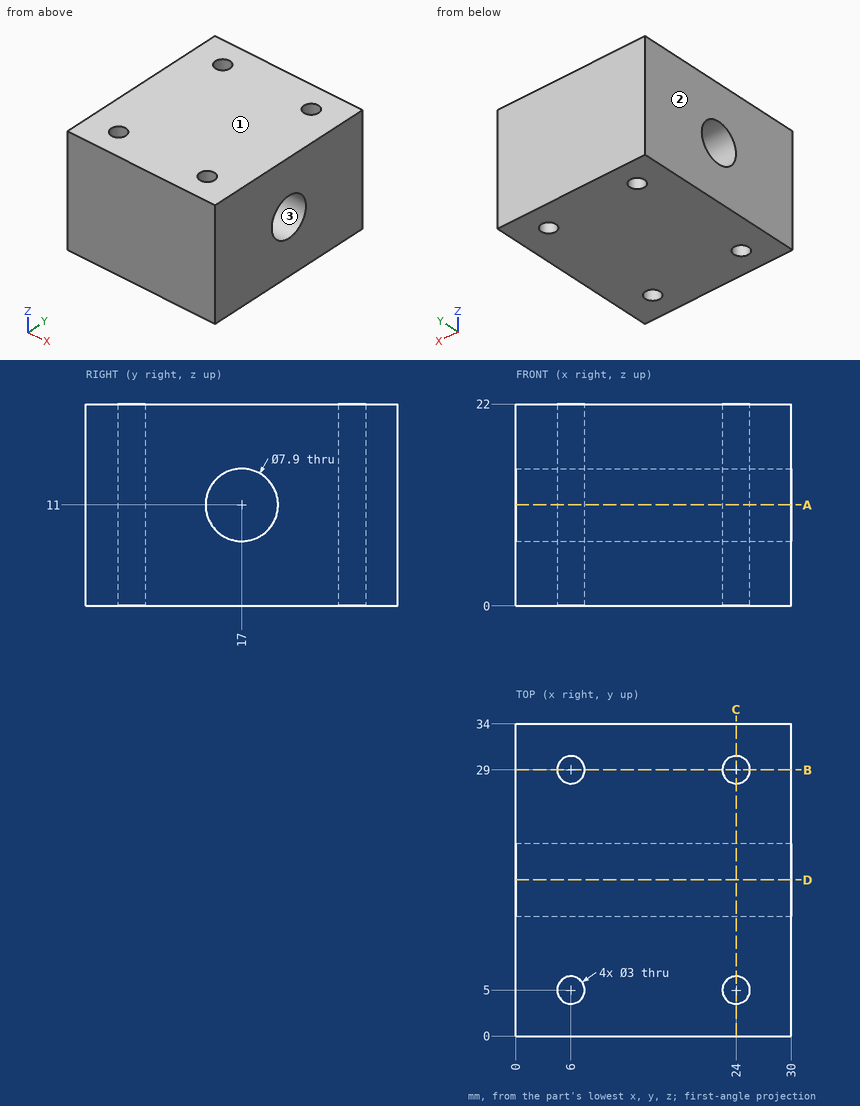
Here's the drawing with two shaded views (mm, measured from the low corner). I have some questions. Give positions to 0.01 mm unless a question says otherwise; leave off trailing zeros. Order: outer loops, then holes, each group sorted by start corner. A loop starts at its lowest first (then second) coordinate and runs counter-clockwise, first axis right, second up. Notation, with made-up numbers: M -40,52.25 L 7,52.25 A32 ccw 7,87.25 Z; hole C 21,57 d3. An arc over 180 degrees is marked long. One line per item, written item: value.
1) I want a section at A-A, the plane z = 11. List the corners of the cut face in (x, y) for me, plus the area to 3 significant figures.
Answer sheet:
outline: M 0,0 L 30,0 L 30,13.05 L 0,13.05 Z; M 0,20.95 L 30,20.95 L 30,34 L 0,34 Z; hole C 6,5 d3; hole C 6,29 d3; hole C 24,5 d3; hole C 24,29 d3
area: 755 mm^2
2) Please list where these lines run through material, in increasing order: line 1 along Y through (x, z) = (24, 6); line 2 along Z through (x, y) = (23, 17); line 3 along Y through (x, z) = (17, 10.75).
Answer sheet:
line 1: y = 0 to 3.5, 6.5 to 27.5, 30.5 to 34
line 2: z = 0 to 7.05, 14.95 to 22
line 3: y = 0 to 13.06, 20.94 to 34
3) I want a section at C-C, the plane x = 24. List the corners of the cut face in (y, z) for me.
Answer sheet:
outline: M 0,0 L 3.5,0 L 3.5,22 L 0,22 Z; M 6.5,0 L 27.5,0 L 27.5,22 L 6.5,22 Z; M 30.5,0 L 34,0 L 34,22 L 30.5,22 Z; hole C 17,11 d7.9
4) For P1, Ø6.5, axis at y = 17, z = 11, coming from the +X side, with a flat end and sliding along its axis, tell me the tip position at first contact or that it passes through.
Answer sheet:
P1: passes through
5) I want a section at B-B, the plane y = 29. List the corners of the cut face in (x, z) for me.
Answer sheet:
outline: M 0,0 L 4.5,0 L 4.5,22 L 0,22 Z; M 7.5,0 L 22.5,0 L 22.5,22 L 7.5,22 Z; M 25.5,0 L 30,0 L 30,22 L 25.5,22 Z
6) We'd pull the mould along Z, two halves only. Please class the marked faces 1, 2 and 3: released by +Z, released by -Z, zero draft, split by the parting line, or undercut.
Answer sheet:
face 1: released by +Z
face 2: zero draft
face 3: undercut
7) I want a section at D-D, the plane y = 17. List the corners of the cut face in (x, z) for me, plus the area to 3 significant figures.
Answer sheet:
outline: M 0,0 L 30,0 L 30,7.05 L 0,7.05 Z; M 0,14.95 L 30,14.95 L 30,22 L 0,22 Z
area: 423 mm^2
